Drawing for the job (mm, zero at the part's lowest x, y, z). A direction names the side the tool comes from. Round coordinates to 2 decimals unless told otherwise and drop trailing zeros. Order: outer loops, then holes, each group sorted by start corner. A loop starts at its lowest first (then second) coordinate and runs counter-clockwise, first axis right, second up. Notation, with made-up numbers: (42.25, 25.5) - (61.25, 25.5) arc R34 cw to (61.25, 63.5) - close; hole circle Ø6 at (39, -34). An arc over 180 degrees is marked (long way). One line per question, with ' | ' between items. Start each with the question number.
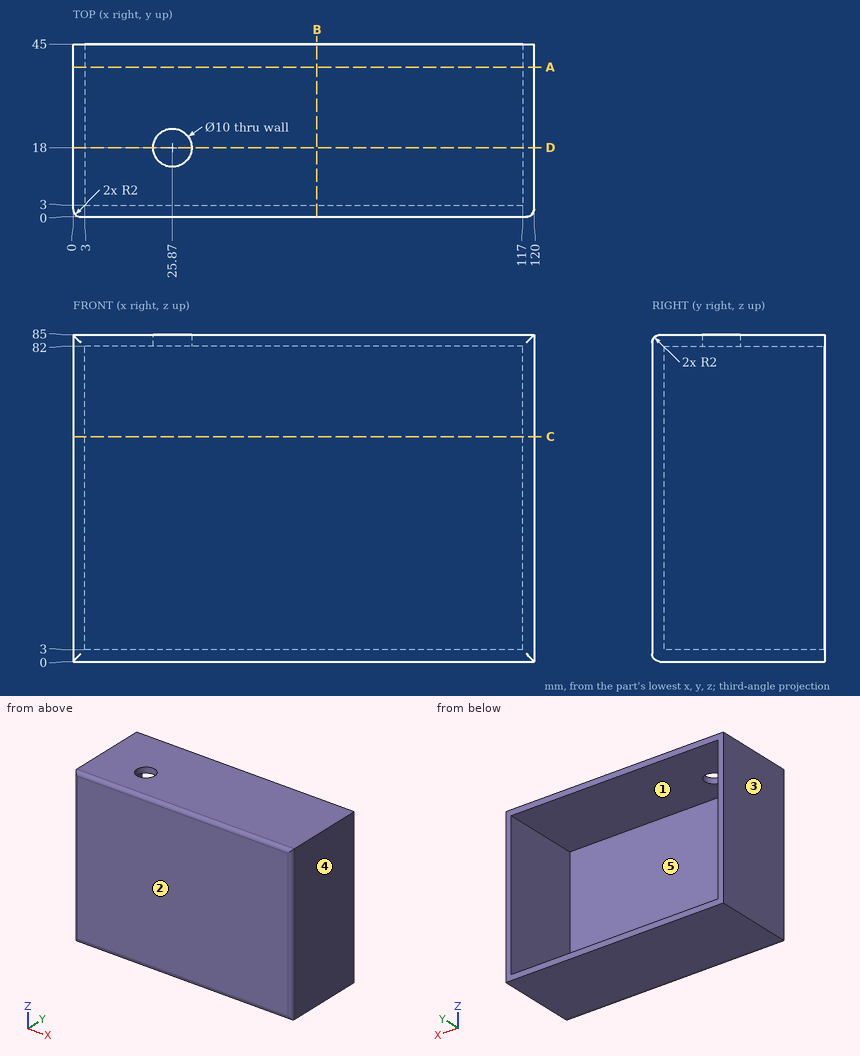
Item 1: Slice it at C-C (z = 58.5). Write the cut outline in (x, y).
Item 2: Wall check: line 1 along Z through (x, y) = (50, 41.5); line 2 along X through (y, z) = (10, 30); line 3 along Y through (x, z) = (28.5, 50.5). Give the ranges that are in metal, low to high. Write a range as [from, to].
Item 3: Slice it at B-B (x = 63.5). Write the cut outline in (y, z).
Item 4: 3-axis set-ups, long thin cutter, end or side, ignore diameter. For the marked faces 4 and 5: which of +Z, -Z, +X, -X, +Y, -Y reach the whole face in a straight line?
Item 5: Pull direction X, two halves, no side cores. Call the marked faces 1, 2 and 3: released by +X, released by -X, zero draft, split by the parting line, or undercut.
Item 6: Slice it at A-A (y = 39). Write the cut outline in (x, z).
Item 7: Slice it at D-D (y = 18). Write the cut outline in (x, z), plus the area to 3 significant figures.
Item 8: Pin check, flat tip, straight feed: pin 1 (23.5 mm diameter, centred on x = 79, z = 49.5, fed in from +Y). Stop position of the tip, or through.
A:
1) outline: (0, 2) arc R2 ccw to (2, 0) - (118, 0) arc R2 ccw to (120, 2) - (120, 45) - (117, 45) - (117, 3) - (3, 3) - (3, 45) - (0, 45) - close
2) line 1: [0, 3], [82, 85] | line 2: [0, 3], [117, 120] | line 3: [0, 3]
3) outline: (0, 2) arc R2 ccw to (2, 0) - (45, 0) - (45, 3) - (3, 3) - (3, 82) - (45, 82) - (45, 85) - (2, 85) arc R2 ccw to (0, 83) - close
4) face 4: +Z, -Z, +X, +Y, -Y | face 5: +Y
5) face 1: undercut | face 2: zero draft | face 3: released by -X
6) outline: (0, 0) - (120, 0) - (120, 85) - (0, 85) - close; hole (3, 3) - (117, 3) - (117, 82) - (3, 82) - close
7) outline: (0, 0) - (120, 0) - (120, 85) - (30.87, 85) - (30.87, 82) - (117, 82) - (117, 3) - (3, 3) - (3, 82) - (20.87, 82) - (20.87, 85) - (0, 85) - close | area: 1,160 mm^2
8) pin 1: y = 3
